Geometry: final body of the model. Coordinates: model frame, mm. Give positions to 0.01 mm unless a question says otherwise; leave off trailing zeros. Write each loop counter-clockwise with the first axis right and the second up, starting at its lowest first coordinate (ties: lowest second). Pieces come first, ordered by that corner, then holes. Notation, with made-up numbers: (29.25, 87.25) - (87.25, 87.25) arc R15 ccw to (87.25, 103.25) - close; hole circle Ø2 at (-39, -27.75). An arc over 180 degrees is marked (long way). Use CSV: the item, a comma, the result in double quotes. Start each with the question number.
(1) Section D-D on z = 2.5. Count the separate pieces of the cut face and the enclosed holes in it, and give its area (3 significant figures).
(2) Section C-C on y = -11. Output: boundary loops of the cut face in (x, z), and give its area (3 significant figures).
(3) Section B-B on x = 41. Output: boundary loops of the cut face in (y, z), and give its area (3 significant figures).
(4) First-contact query: pin 1 Ø1.2 at (x, z) = (0, 2) entering from -Y; pin 2 Ø1.2 at (x, z) = (22, 1.5) entering from +Y; pin 3 Ø7 at (x, y) = (41, -10) entering from -Z. Flat tips, straight axial feed; report the tip coordinate or a pass-through.
(5) Line query: probe 1 along Y at (x, z) = (41, 2.7); probe 2 along X at (y, z) = (0, 1.2); probe 3 along X at (y, z) = (4, 0.6). Output: solid intervals per line, ascending. Write a range as [from, to].
(6) Section A-A on x = -6. Output: boundary loops of the cut face in (y, z), and give its area (3 significant figures).
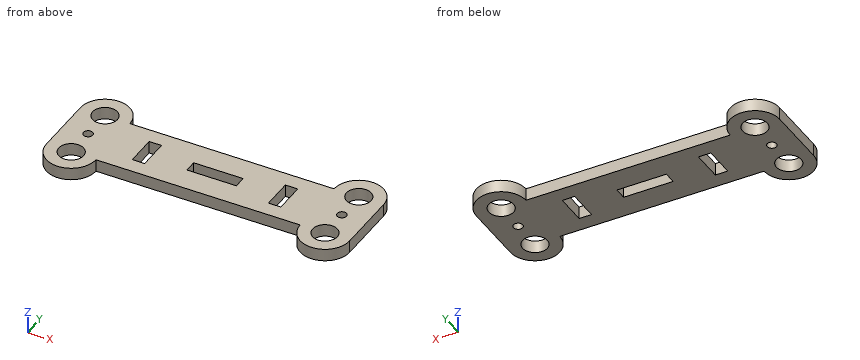
Autodesk Inventor part; units mm, degrees
ref_plane "YZ Plane" through (0, 0, 0) normal (1, 0, 0) x (0, 1, 0)
ref_plane "XZ Plane" through (0, 0, 0) normal (0, 1, 0) x (-1, 0, 0)
ref_plane "XY Plane" through (0, 0, 0) normal (0, 0, 1) x (1, 0, 0)
sketch "Эскиз1" plane through (0, 0, 0) normal (0, 0, 1) x (1, 0, 0)
  circle A0 centre (-41, -10) radius 4
  circle A1 centre (-41, 10) radius 4
  circle A2 centre (41, 10) radius 4
  circle A3 centre (41, -10) radius 4
  line L0 (-41, 10) -> (41, 10) construction
  line L1 (41, 10) -> (41, -10) construction
  line L2 (41, -10) -> (-41, -10) construction
  line L3 (-41, -10) -> (-41, 10) construction
  arc A4 (-33, 10) -> (-49, 10) centre (-41, 10) ccw
  arc A5 (-49, -10) -> (-33, -10) centre (-41, -10) ccw
  arc A6 (33, -10) -> (49, -10) centre (41, -10) ccw
  arc A7 (49, 10) -> (33, 10) centre (41, 10) ccw
  line L4 (-49, 10) -> (-49, -10)
  line L5 (49, 10) -> (49, -10)
  line L6 (33, 10) -> (-33, 10)
  line L7 (33, -10) -> (-33, -10)
  line L8 (8, -2) -> (-8, -2)
  line L9 (-8, -2) -> (-8, 2)
  line L10 (-8, 2) -> (8, 2)
  line L11 (8, 2) -> (8, -2)
  line L12 (24, 5) -> (20, 5)
  line L13 (20, 5) -> (20, -5)
  line L14 (20, -5) -> (24, -5)
  line L15 (24, -5) -> (24, 5)
  line L16 (0, 10) -> (0, -10)
  line L17 (-24, 5) -> (-20, 5)
  line L18 (-20, 5) -> (-20, -5)
  line L19 (-20, -5) -> (-24, -5)
  line L20 (-24, -5) -> (-24, 5)
  point P0 (0, 0)
  point P1 (41, 0)
  point P2 (0, 2)
  point P3 (8, 0)
  point P4 (20, 0)
  point P5 (-20, 0)
  dimension "d0" = 8
  dimension "d1" = 20
  dimension "d2" = 82
  dimension "d3" = 8
  dimension "d6" = 10
  dimension "d7" = 10
  dimension "d8" = 4
  dimension "d9" = 16
  dimension "d10" = 10
  dimension "d11" = 40
extrude "Выдавливание1" add sketch "Эскиз1" along normal blind 4 contours L6 L16 L10 L9 L8 L7 A5 L4 A4 | L6 A7 L5 A6 L7 L16 L8 L11 L10
sketch "Эскиз2" plane through (0, 0, 4) normal (0, 0, 1) x (1, 0, 0)
  line L0 (-8, -2) -> (-8, 2)
  line L1 (-8, 2) -> (8, 2)
  line L2 (8, 2) -> (8, -2)
  line L3 (8, -2) -> (-8, -2)
  circle A0 centre (41, -10) radius 4
  circle A1 centre (41, 10) radius 4
  circle A2 centre (-41, 10) radius 4
  circle A3 centre (-41, -10) radius 4
  line L4 (-20, 5) -> (-20, -5)
  line L5 (-20, -5) -> (-24, -5)
  line L6 (-24, -5) -> (-24, 5)
  line L7 (-24, 5) -> (-20, 5)
  line L8 (24, 5) -> (24, -5)
  line L9 (24, -5) -> (20, -5)
  line L10 (20, -5) -> (20, 5)
  line L11 (20, 5) -> (24, 5)
  arc A4 (-33, 10) -> (-49, 10) centre (-41, 10) ccw
  line L12 (-49, 10) -> (-49, -10)
  arc A5 (-49, -10) -> (-33, -10) centre (-41, -10) ccw
  line L13 (-33, -10) -> (33, -10)
  arc A6 (33, -10) -> (49, -10) centre (41, -10) ccw
  line L14 (49, -10) -> (49, 10)
  arc A7 (49, 10) -> (33, 10) centre (41, 10) ccw
  line L15 (33, 10) -> (-33, 10)
  point P0 (0, 0)
  point P1 (41, 0)
  point P2 (-41, 0)
hole "Отверстие1" at (41, 0, 4) at (-41, 0, 4) direction (0, 0, -1) diameter 3 end through all
properties part number "PistonPart1" material "Дерево (вишня)"
Check values:
1,separate pieces,"1"
1,enclosed holes,"9"
1,area,"2,000 mm²"
2,outline,"(-48.94, 0) - (-44.87, 0) - (-44.87, 4) - (-48.94, 4) - close; (-37.13, 0) - (-33.06, 0) - (-33.06, 4) - (-37.13, 4) - close; (33.06, 0) - (37.13, 0) - (37.13, 4) - (33.06, 4) - close; (44.87, 0) - (48.94, 0) - (48.94, 4) - (44.87, 4) - close"
2,area,"65.0 mm²"
3,outline,"(-18, 0) - (-14, 0) - (-14, 4) - (-18, 4) - close; (-6, 0) - (-1.5, 0) - (-1.5, 4) - (-6, 4) - close; (1.5, 0) - (6, 0) - (6, 4) - (1.5, 4) - close; (14, 0) - (18, 0) - (18, 4) - (14, 4) - close"
3,area,"68.0 mm²"
4,pin 1,"stops at y = -10"
4,pin 2,"stops at y = 10"
4,pin 3,"passes through"
5,probe 1,"y = [-18, -14], [-6, -1.5], [1.5, 6], [14, 18]"
5,probe 2,"x = [-49, -42.5], [-39.5, -24], [-20, -8], [8, 20], [24, 39.5], [42.5, 49]"
5,probe 3,"x = [-49, -24], [-20, 20], [24, 49]"
6,outline,"(-10, 0) - (-2, 0) - (-2, 4) - (-10, 4) - close; (2, 0) - (10, 0) - (10, 4) - (2, 4) - close"
6,area,"64.0 mm²"
